from build123d import *

# Parameters (mm, degrees)
SALIENTE_EXTRUIR1_DEPTH = 0.1


with BuildPart() as part:
    # Model → Saliente-Extruir1 (new body)
    with BuildSketch(Plane.XY):
        with BuildLine():
            Line((29.512585392, 24.480394017), (27.703067566, 39.527605983))
            ThreePointArc((27.703067566, 39.527605983), (7.377127931, 35.592311556), (-10.673926914, 25.453781916))
            ThreePointArc((-10.673926914, 25.453781916), (-10.212179423, 19.928358371), (-8.854222662, 14.552535688))
            ThreePointArc((-8.854222662, 14.552535688), (-3.021164415, 16.754836825), (2.933605753, 18.6029199))
            Line((2.933605753, 18.6029199), (19.512585392, 31.480394017))
            Line((19.512585392, 31.480394017), (24.573492595, 10.397787824))
            Line((24.573492595, 10.397787824), (39.831918887, 14.06059302))
            Line((39.831918887, 14.06059302), (45.938881991, 27.30453113))
            Line((45.938881991, 27.30453113), (29.512585392, 24.480394017))
        make_face()
    extrude(amount=SALIENTE_EXTRUIR1_DEPTH)


solid = part.part
Geometry: final body of the model. Coordinates: model frame, mm. Give positions to 0.01 mm unless a question says otherwise; leave off trailing zeros. Order: outer loops, then holes, each group sorted by start corner. A loop starts at its lowest first (then second) coordinate and runs counter-clockwise, first axis right, second up. Notation, with made-up numbers: (88, 88.5) -> (120, 88.5) arc R13 ccw to (120, 107.5) -> close; hole circle Ø5 at (59.25, 58). An arc over 180 degrees is marked (long way). Put each result on its own line as item: value.
Q1. Material intervals for L1, parallel to Y at x = 14, z = 0.05; L2, parallel to Y at x = 13, z = 0.05, sorted ascending.
Here are the results:
L1: y = 27.2 to 37.63
L2: y = 26.42 to 37.37
Q2. Section D-D, the plane x = 34.5. Return loops of the section in (y, z).
Here are the results:
outline: (12.78, 0) -> (25.34, 0) -> (25.34, 0.1) -> (12.78, 0.1) -> close
Q3. Section C-C, the plane y = 16. Return loops of the section in (x, z).
Here are the results:
outline: (-9.31, 0) -> (-5.14, 0) -> (-5.14, 0.1) -> (-9.31, 0.1) -> close; (23.23, 0) -> (40.73, 0) -> (40.73, 0.1) -> (23.23, 0.1) -> close
Q4. Section B-B, the plane y = 20. Return loops of the section in (x, z).
Here are the results:
outline: (-10.22, 0) -> (4.73, 0) -> (4.73, 0.1) -> (-10.22, 0.1) -> close; (22.27, 0) -> (42.57, 0) -> (42.57, 0.1) -> (22.27, 0.1) -> close
Q5. Section A-A, the plane z = 0.05. Return loops of the section in (x, y).
Here are the results:
outline: (-10.67, 25.45) arc R33.84 ccw to (-8.85, 14.55) arc R103.79 cw to (2.93, 18.6) -> (19.51, 31.48) -> (24.57, 10.4) -> (39.83, 14.06) -> (45.94, 27.3) -> (29.51, 24.48) -> (27.7, 39.53) arc R64.87 ccw to start
